from build123d import *

# Parameters (mm, degrees)
SKETCH3_W           = 160
SKETCH3_H           = 250
BOSS_EXTRUDE2_DEPTH = 1.5
SKETCH4_R           = 5
CUT_EXTRUDE4_DEPTH  = 149.415801046
SKETCH6_W           = 1.5
SKETCH6_H           = 190
BOSS_EXTRUDE4_DEPTH = 45


with BuildPart() as part:
    # Sketch3 → Boss-Extrude2 (new body)
    with BuildSketch(Plane.XY):
        Rectangle(SKETCH3_W, SKETCH3_H)
    extrude(amount=BOSS_EXTRUDE2_DEPTH)

    # Sketch4 → Cut-Extrude4 (cut, through all)
    with BuildSketch(Plane.XY):
        with Locations((-11.69, -66.6)):
            Circle(SKETCH4_R)
    extrude(amount=CUT_EXTRUDE4_DEPTH, mode=Mode.SUBTRACT)

    # Sketch6 → Boss-Extrude4 (add)
    with BuildSketch(Plane.XY.offset(1.5)):
        Polygon((-73.5, 13.5), (-73.5, 125), (-75, 125), (-75, -125), (-73.5, -125), align=None)
        with Locations((74.25, 30)):
            Rectangle(SKETCH6_W, SKETCH6_H)
    extrude(amount=BOSS_EXTRUDE4_DEPTH)


solid = part.part
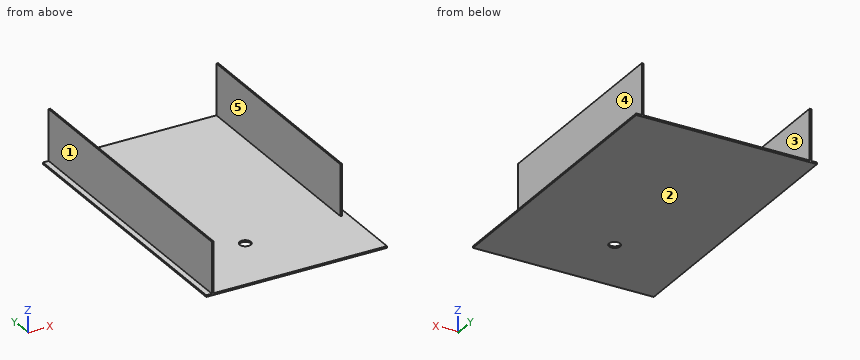
Geometry: final body of the model. Coordinates: model frame, mm. Face numbers are marked on the shaded views. A direction names the side the tool comes from. Give positions to 0.01 mm unless a question says otherwise; leave off trailing zeros. Write each loop counter-clockwise with the first axis right and the second up, starting at its lowest first coordinate (ties: lowest second). Pieces come first, ordered by that corner, then holes.
(1) Ray query, line 1 (X direction, y = 58, z = 3); line 2 (Y direction, x = -11.69, z = 0.4); line 3 (X direction, y = -66.6, z = 0.55). Return the intervals inside material, ascending.
(2) Access query for the marked faces 4 and 5. Directions: +Z, -Z, +X, -X, +Y, -Y. A direction counts if a zero-diameter tool reaches every point of the face in a straight line with its end or side. Return the directions, or none.
(3) Mould query, pull axis X, two halves, no side actions, for the marked faces 1, 2 and 3. Classes: released by +X, released by -X, zero draft, split by the parting line, or undercut.
(4) Cut plane D-D, the plane y = 23. Return loops of the section in (x, z), then the cut area to 3 significant figures.
(5) Cut plane C-C, the plane y = -100. Return loops of the section in (x, z).
(6) Cut plane B-B, the plane z = 29.5. Return loops of the section in (x, y), then the cut area to 3 significant figures.
(7) Cut plane A-A, the plane x = -11.69. Return loops of the section in (y, z), then the cut area to 3 significant figures.
(8) First-contact query: P1, Ø6, axis at y = -68.5, z = 22, coming from the -X side; P2, Ø1.6, axis at x = 74.5, z = 31.5, coming from the -Y side; P3, Ø13.5, axis at y = 7.5, z = 28.5, coming from the +X side. Flat tips, straight axial feed; report the tip coordinate or a pass-through.
Values follow:
1. line 1: x = -75 to -73.5, 73.5 to 75
1. line 2: y = -125 to -71.6, -61.6 to 125
1. line 3: x = -80 to -16.69, -6.69 to 80
2. face 4: +Z, +X, +Y, -Y
2. face 5: +Z, +Y, -Y
3. face 1: released by -X
3. face 2: zero draft
3. face 3: undercut
4. outline: (-80, 0) - (80, 0) - (80, 1.5) - (75, 1.5) - (75, 46.5) - (73.5, 46.5) - (73.5, 1.5) - (-73.5, 1.5) - (-73.5, 46.5) - (-75, 46.5) - (-75, 1.5) - (-80, 1.5) - close
4. area: 375 mm2
5. outline: (-80, 0) - (80, 0) - (80, 1.5) - (-73.5, 1.5) - (-73.5, 46.5) - (-75, 46.5) - (-75, 1.5) - (-80, 1.5) - close
6. outline: (-75, -125) - (-73.5, -125) - (-73.5, 125) - (-75, 125) - close; (73.5, -65) - (75, -65) - (75, 125) - (73.5, 125) - close
6. area: 660 mm2
7. outline: (-125, 0) - (-71.6, 0) - (-71.6, 1.5) - (-125, 1.5) - close; (-61.6, 0) - (125, 0) - (125, 1.5) - (-61.6, 1.5) - close
7. area: 360 mm2
8. P1: stops at x = -75
8. P2: stops at y = -65
8. P3: stops at x = 75
